The drawing under review shows one solid part. Ordinate dimensions are in mm from its lowest x, y, z. A direction names the side the tool comes from. Give positions to 0.01 mm unless a question says otherwise; leave off trailing zeros. Write each loop counter-clockwise with the first axis right and the second up, starting at its lowest first coordinate (ties: lowest second). Pieces come first, ordered by that corner, then holes. Notation, with made-up numbers: M 52.5,10 L 69.5,10 A22 cw 69.5,43 Z; hole C -21,0.5 d2. An arc over 180 degrees is marked long. One line per item, written item: value. Start each with the question number.
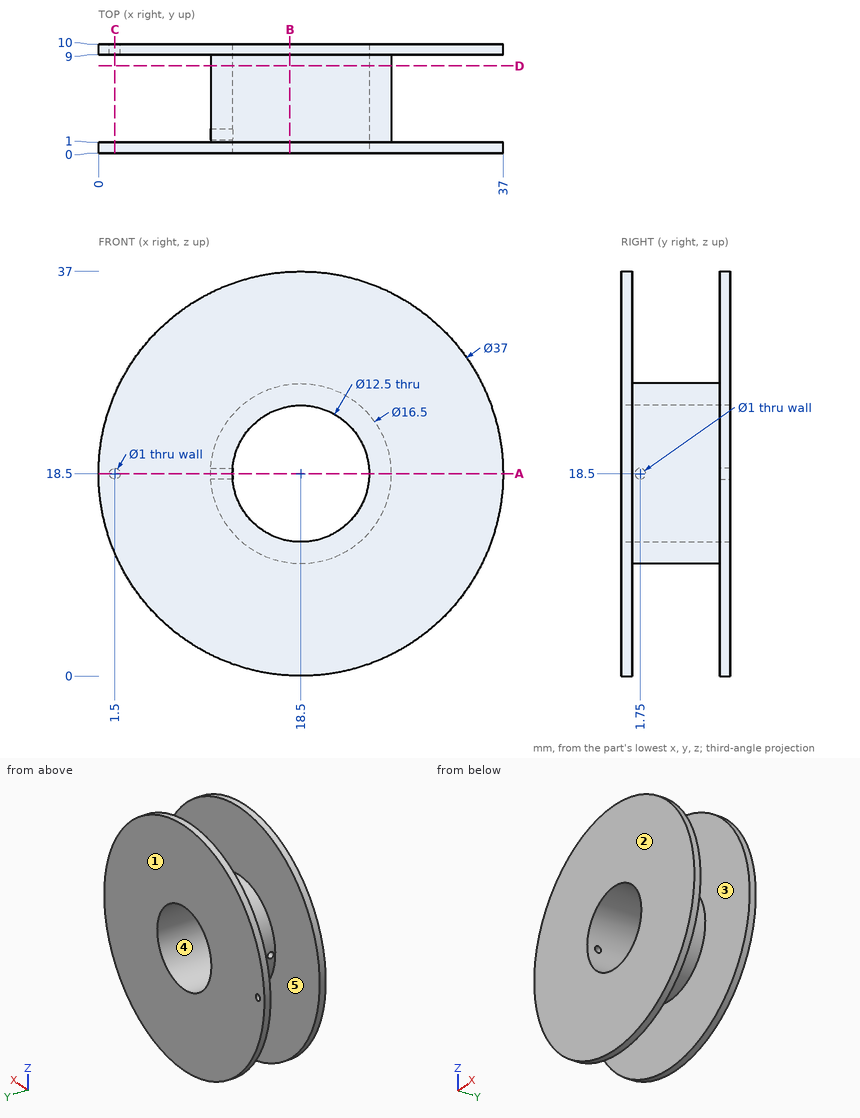
Q1. For P1, Ø1, axis at x = 12.5, y = 7.5, coming from the -Z side; P2, Ø3, axis at x = 15, y = 9, coming from the -Z side; P3, Ø2, axis at x = 24, y = 9, coming from the -Z side, all flat-tipped, find the tip position at first contact; note any pin that passes through.
Q2. Take a section at B-B, the plane x = 17.5. Give the boundary of the cut face in (y, z).
Q3. Machinability: for the marked faces 4 and 5, which of the approach directions +Z, -Z, +X, -X, +Y, -Y give a long, thin tool a straight path to every point of the face, cutting with its end or side? Answer none if there is none.
Q4. Take a section at D-D, the plane y = 8. Give the boundary of the cut face in (x, z), then the cut area to 3 significant figures.
Q5. Take a section at A-A, the plane z = 18.5. Give the boundary of the cut face in (x, y), then the cut area to 3 significant figures.
Q6. Wall thickness on line 1 (X direction, y = 9.3, z = 18.5); line 2 (Y direction, x = 4, z = 27.5); line 3 (X direction, y = 3.25, z = 18.5): over which ranges is each line inside the solid? List them lowest first. Write a range as from..to.
Q7. Take a section at C-C, the plane x = 1.5. Give the boundary of the cut face in (y, z).
Q8. The part is to be moulded in two halves that separate along Y. For the marked faces 1, 2 and 3, say which applies: pulls with the +Y half, pulls with the -Y half, needs draft (parallel to the pull), parting line crosses it, or undercut.
Results list:
1. P1: stops at z = 12.35
1. P2: stops at z = 0.11
1. P3: stops at z = 0.56
2. outline: M 0,0.03 L 1,0.03 L 1,10.31 L 9,10.31 L 9,0.03 L 10,0.03 L 10,12.33 L 0,12.33 Z; M 0,24.67 L 10,24.67 L 10,36.97 L 9,36.97 L 9,26.69 L 1,26.69 L 1,36.97 L 0,36.97 Z
3. face 4: +Y, -Y
3. face 5: none
4. outline: C 18.5,18.5 d16.5; hole C 18.5,18.5 d12.5
4. area: 91.1 mm^2
5. outline: M 0,0 L 12.25,0 L 12.25,1.25 L 10.25,1.25 L 10.25,1 L 0,1 Z; M 0,9 L 1,9 L 1,10 L 0,10 Z; M 2,9 L 10.25,9 L 10.25,2.25 L 12.25,2.25 L 12.25,10 L 2,10 Z; M 24.75,0 L 37,0 L 37,1 L 26.75,1 L 26.75,9 L 37,9 L 37,10 L 24.75,10 Z
5. area: 78.0 mm^2
6. line 1: x = 0..1, 2..12.25, 24.75..37
6. line 2: y = 0..1, 9..10
6. line 3: x = 10.25..12.25, 24.75..26.75
7. outline: M 0,11.2 L 1,11.2 L 1,25.8 L 0,25.8 Z; M 9,11.2 L 10,11.2 L 10,18 L 9,18 Z; M 9,19 L 10,19 L 10,25.8 L 9,25.8 Z
8. face 1: pulls with the +Y half
8. face 2: pulls with the -Y half
8. face 3: undercut
